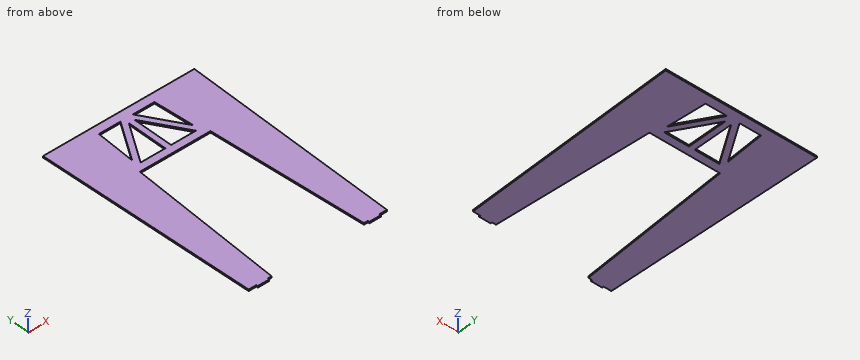
```python
from build123d import *

# Parameters (mm, degrees)
BOSS_EXTRUDE1_DEPTH = 10.16
CUT_EXTRUDE1_DEPTH  = 12.7


with BuildPart() as part:
    # Sketch1 → Boss-Extrude1 (new body)
    with BuildSketch(Plane.XY):
        Polygon((-502.783260533, 1465.163333881), (-459.721789204, 17.476365817), (-408.921789204, 17.476365817), (-408.921789204, 7.316365817), (-332.100796745, 7.316365817), (-332.100796745, 17.476365817), (-306.627827519, 17.476365817), (-234.627172097, 1054.1), (234.627172097, 1054.1), (306.627827519, 17.476365817), (332.721789204, 17.476365817), (332.721789204, 7.316365817), (408.921789204, 7.316365817), (408.921789204, 17.476365817), (459.721789204, 17.476365817), (502.783260533, 1465.163333881), align=None)
        Polygon((183.241684323, 1104.9), (19.05, 1104.9), (19.05, 1370.513438368), align=None, mode=Mode.SUBTRACT)
        Polygon((-184.672467887, 1406.743333881), (-41.445883295, 1406.743333881), (-202.80261453, 1145.716008632), align=None, mode=Mode.SUBTRACT)
        Polygon((-19.05, 1370.513438368), (-19.05, 1104.9), (-183.241684323, 1104.9), align=None, mode=Mode.SUBTRACT)
        Polygon((184.672467887, 1406.743333881), (202.80261453, 1145.716008632), (41.445883295, 1406.743333881), align=None, mode=Mode.SUBTRACT)
    extrude(amount=BOSS_EXTRUDE1_DEPTH)

    # Sketch2 → Cut-Extrude1 (cut)
    with BuildSketch(Plane.XY):
        Polygon((271.312390408, 664.982386142), (264.796190418, 758.798850391), (254.678510334, 758.096107781), (261.194710324, 664.279643533), align=None)
        Polygon((283.630301787, 487.636249721), (277.115944656, 581.426181539), (266.998264572, 580.72343893), (273.512621703, 486.933507112), align=None)
        Polygon((295.948213166, 310.290113301), (289.435698895, 404.053512688), (279.318018811, 403.350770078), (285.830533081, 309.587370692), align=None)
        Polygon((308.266124544, 132.94397688), (301.755453134, 226.680843836), (291.63777305, 225.978101227), (298.14844446, 132.241234271), align=None)
        Polygon((-301.755453134, 226.680843836), (-308.266124544, 132.94397688), (-298.14844446, 132.241234271), (-291.63777305, 225.978101227), align=None)
        Polygon((-289.435698895, 404.053512688), (-295.948213166, 310.290113301), (-285.830533081, 309.587370692), (-279.318018811, 403.350770078), align=None)
        Polygon((-277.115944656, 581.426181539), (-283.630301787, 487.636249721), (-273.512621703, 486.933507112), (-266.998264572, 580.72343893), align=None)
        Polygon((-264.796190418, 758.798850391), (-271.312390408, 664.982386142), (-261.194710324, 664.279643533), (-254.678510334, 758.096107781), align=None)
    extrude(amount=-CUT_EXTRUDE1_DEPTH, mode=Mode.SUBTRACT)


solid = part.part
```
Model file for the job. Use its own axes, mm. Give positions to 0.01 mm unless a question says otherwise; leave off trailing zeros. Write each loop counter-clockwise with the first axis right and the second up, starting at its lowest first coordinate (ties: lowest second). Pieces come first, ordered by that corner, then holes. Notation, with made-up numbers: (81, 50) - (108, 50) arc R19 ccw to (108, 83) - close; hole circle Ø3 at (65, 50.5). An arc over 180 degrees is marked (long way). One line per question, with ' | ' between items. Start each with the question number.
(1) Wall check: line 1 along Y through (x, z) = (-171.5, 0.75); line 2 along X through (y, z) = (1253, 4.25); line 3 along Y through (x, z) = (-7, 6.5). Give the ranges that are in metal, low to high. Write a range as from..to.
(2) Pin check, flat tips, straight feed: P1, Ø3, axis at x = -107.5, z = 5.5, coming from the -Y side; P2, Ø3, axis at x = 439, z = 3.5, coming from the -Y side; P3, Ø3, axis at y = 1270, z = 6.5, coming from the +X side; P4, Ø1, axis at x = -393.5, y = 679.5, coming from the -Z side. Stop position of each tip, or through.
(3) Slice it at D-D on y = 1338. Write the cut outline in (x, z), plus the area to 3 significant figures.
(4) Slice it at C-C on y = 940.5. Write the cut outline in (x, z), plus the area to 3 significant figures.
(5) Slice it at B-B on x = 56. Write the cut outline in (y, z).
(6) Slice it at A-A on z = 6.5. Write the cut outline in (x, y), plus the area to 3 significant figures.
Results below:
1) line 1: 1054.1..1104.9, 1123.89..1196.35, 1406.74..1465.16 | line 2: -496.47..-195.35, -136.48..-91.69, -19.05..19.05, 91.69..136.48, 195.35..496.47 | line 3: 1054.1..1465.16
2) P1: y = 1054.1 | P2: y = 17.48 | P3: x = 497.02 | P4: z = 0
3) outline: (-499, 0) - (-189.45, 0) - (-189.45, 10.16) - (-499, 10.16) - close; (-83.94, 0) - (-39.15, 0) - (-39.15, 10.16) - (-83.94, 10.16) - close; (-19.05, 0) - (19.05, 0) - (19.05, 10.16) - (-19.05, 10.16) - close; (39.15, 0) - (83.94, 0) - (83.94, 10.16) - (39.15, 10.16) - close; (189.45, 0) - (499, 0) - (499, 10.16) - (189.45, 10.16) - close | area: 7,590 mm^2
4) outline: (-487.18, 0) - (-242.52, 0) - (-242.52, 10.16) - (-487.18, 10.16) - close; (242.52, 0) - (487.18, 0) - (487.18, 10.16) - (242.52, 10.16) - close | area: 4,970 mm^2
5) outline: (1054.1, 0) - (1104.9, 0) - (1104.9, 10.16) - (1054.1, 10.16) - close; (1310.74, 0) - (1383.2, 0) - (1383.2, 10.16) - (1310.74, 10.16) - close; (1406.74, 0) - (1465.16, 0) - (1465.16, 10.16) - (1406.74, 10.16) - close
6) outline: (-502.78, 1465.16) - (-459.72, 17.48) - (-408.92, 17.48) - (-408.92, 7.32) - (-332.1, 7.32) - (-332.1, 17.48) - (-306.63, 17.48) - (-234.63, 1054.1) - (234.63, 1054.1) - (306.63, 17.48) - (332.72, 17.48) - (332.72, 7.32) - (408.92, 7.32) - (408.92, 17.48) - (459.72, 17.48) - (502.78, 1465.16) - close; hole (-202.8, 1145.72) - (-41.45, 1406.74) - (-184.67, 1406.74) - close; hole (-183.24, 1104.9) - (-19.05, 1104.9) - (-19.05, 1370.51) - close; hole (19.05, 1104.9) - (183.24, 1104.9) - (19.05, 1370.51) - close; hole (41.45, 1406.74) - (202.8, 1145.72) - (184.67, 1406.74) - close | area: 753,000 mm^2
